from build123d import *

# Parameters (mm, degrees)
F0_W      = 155.180738
F0_H      = 90
F1_DEPTH  = 25
F2_R      = 16.845897
F3_DEPTH  = 25.001
F1_FACE_W = 155.180738
F1_FACE_H = 90
F1_FACE_R = 16.845897
F4_DEPTH  = 50


with BuildPart() as f1:
    # F0 (on Front) → F1 (new body)
    with BuildSketch(Plane.XZ):
        with Locations((27.717258, -13.581821)):
            Rectangle(F0_W, F0_H)
    extrude(amount=F1_DEPTH)

    # F2 (on face) → F3 (cut, through all)
    with BuildSketch(Plane.XZ.offset(25)):
        with Locations((13.070613, 0)):
            Circle(F2_R)
    extrude(amount=-F3_DEPTH, mode=Mode.SUBTRACT)

    # F1_face (on face) → F4 (join)
    with BuildSketch(Plane(origin=(27.717258, -25, -13.581821), x_dir=(1, 0, 0), z_dir=(0, -1, 0))):
        Rectangle(F1_FACE_W, F1_FACE_H)
        with Locations((-14.646645, 13.581821)):
            Circle(F1_FACE_R, mode=Mode.SUBTRACT)
    extrude(amount=F4_DEPTH)


solid = f1.part
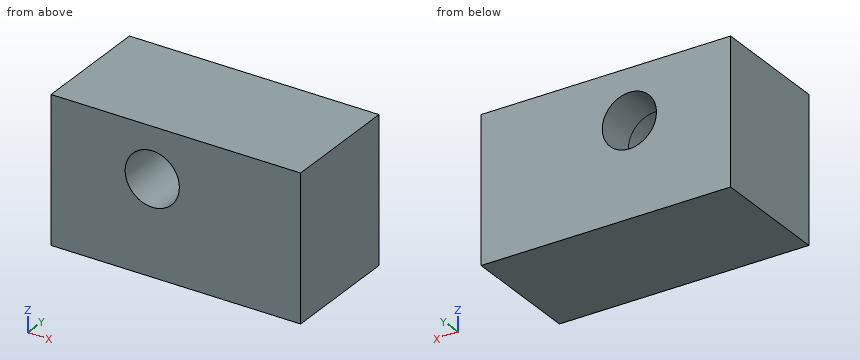
Source: CAD feature listing. Evaluate the final solid. Frame: model axes, mm. Round coordinates to 2 decimals unless told otherwise and drop trailing zeros. Loops run counter-clockwise (first coordinate to the right, second up) from the corner with the lowest first, then second, coordinate; pieces in that order, holes last. Notation, with made-up numbers: (-19, 40.25) -> (4, 40.25) arc R18 cw to (4, 54.25) -> close; hole circle Ø11 at (36, 25.5). An arc over 180 degrees is marked (long way). Answer as a JSON object with one key per item and string values. Group by question number.
Q1. Ray query, line 1 (X direction, y = -8.5, z = 9); line 2 (Z direction, x = 23, y = -4); line 3 (X direction, y = -19, z = 7.5). Return the intervals inside material, ascending. Write a range as from..to.
Q2. Section query B-B (x = 23). Output: boundary loops of the cut face in (y, z).
Q3. Section query C-C (y = -6.5). Output: boundary loops of the cut face in (x, z).
Q4. Section query A-A (z = 0). Output: boundary loops of the cut face in (x, y).
Completed:
{
 "1": {"line 1": "-49.87..-1.17, 27.31..105.31", "line 2": "-58.58..-13.61, 13.61..31.42", "line 3": "-49.87..-2.01, 28.15..105.31"},
 "2": {"outline": "(-75, -58.58) -> (0, -58.58) -> (0, -13.61) -> (-75, -13.61) -> close; (-75, 13.61) -> (0, 13.61) -> (0, 31.42) -> (-75, 31.42) -> close"},
 "3": {"outline": "(-49.87, -58.58) -> (105.31, -58.58) -> (105.31, 31.42) -> (-49.87, 31.42) -> close; hole circle Ø33.69 at (13.07, 0)"},
 "4": {"outline": "(-49.87, -75) -> (-3.78, -75) -> (-3.78, 0) -> (-49.87, 0) -> close; (29.92, -75) -> (105.31, -75) -> (105.31, 0) -> (29.92, 0) -> close"}
}
